from build123d import *

# Parameters (mm, degrees)
SKETCH_1_R      = 2.5
EXTRUDE_1_DEPTH = 140


with BuildPart() as part:
    # 草图1 → 凸台-拉伸1 (new, symmetric)
    with BuildSketch(Plane(origin=(0, 0, 0), x_dir=(1, 0, 0), z_dir=(0, 1, 0))):
        with BuildLine():
            Line((15.752176799, 53.551974455), (15.752176799, 48.473294799))
            Line((15.752176799, 48.473294799), (12.791516627, 45.512634627))
            Line((12.791516627, 45.512634627), (11.152176799, 45.512634627))
            Line((11.152176799, 45.512634627), (11.152176799, 47.912634627))
            Line((11.152176799, 47.912634627), (10.152176799, 47.912634627))
            Line((10.152176799, 47.912634627), (10.152176799, 47.412634627))
            Line((10.152176799, 47.412634627), (9.352176799, 47.412634627))
            Line((9.352176799, 47.412634627), (9.352176799, 42.512634627))
            ThreePointArc((9.352176799, 42.512634627), (9.791516627, 41.451974455), (10.852176799, 41.012634627))
            Line((10.852176799, 41.012634627), (15.752176799, 41.012634627))
            Line((15.752176799, 41.012634627), (15.752176799, 41.812634627))
            Line((15.752176799, 41.812634627), (16.252176799, 41.812634627))
            Line((16.252176799, 41.812634627), (16.252176799, 42.812634627))
            Line((16.252176799, 42.812634627), (13.852176799, 42.812634627))
            Line((13.852176799, 42.812634627), (13.852176799, 44.451974455))
            Line((13.852176799, 44.451974455), (16.812836971, 47.412634627))
            Line((16.812836971, 47.412634627), (21.891516627, 47.412634627))
            Line((21.891516627, 47.412634627), (24.852176799, 44.451974455))
            Line((24.852176799, 44.451974455), (24.852176799, 42.812634627))
            Line((24.852176799, 42.812634627), (22.452176799, 42.812634627))
            Line((22.452176799, 42.812634627), (22.452176799, 41.812634627))
            Line((22.452176799, 41.812634627), (22.952176799, 41.812634627))
            Line((22.952176799, 41.812634627), (22.952176799, 41.012634627))
            Line((22.952176799, 41.012634627), (27.852176799, 41.012634627))
            ThreePointArc((27.852176799, 41.012634627), (28.912836971, 41.451974455), (29.352176799, 42.512634627))
            Line((29.352176799, 42.512634627), (29.352176799, 47.412634627))
            Line((29.352176799, 47.412634627), (28.552176799, 47.412634627))
            Line((28.552176799, 47.412634627), (28.552176799, 47.912634627))
            Line((28.552176799, 47.912634627), (27.552176799, 47.912634627))
            Line((27.552176799, 47.912634627), (27.552176799, 45.512634627))
            Line((27.552176799, 45.512634627), (25.912836971, 45.512634627))
            Line((25.912836971, 45.512634627), (22.952176799, 48.473294799))
            Line((22.952176799, 48.473294799), (22.952176799, 53.551974455))
            Line((22.952176799, 53.551974455), (25.912836971, 56.512634627))
            Line((25.912836971, 56.512634627), (27.552176799, 56.512634627))
            Line((27.552176799, 56.512634627), (27.552176799, 54.112634627))
            Line((27.552176799, 54.112634627), (28.552176799, 54.112634627))
            Line((28.552176799, 54.112634627), (28.552176799, 54.612634627))
            Line((28.552176799, 54.612634627), (29.352176799, 54.612634627))
            Line((29.352176799, 54.612634627), (29.352176799, 59.512634627))
            ThreePointArc((29.352176799, 59.512634627), (28.912836971, 60.573294799), (27.852176799, 61.012634627))
            Line((27.852176799, 61.012634627), (22.952176799, 61.012634627))
            Line((22.952176799, 61.012634627), (22.952176799, 60.212634627))
            Line((22.952176799, 60.212634627), (22.452176799, 60.212634627))
            Line((22.452176799, 60.212634627), (22.452176799, 59.212634627))
            Line((22.452176799, 59.212634627), (24.852176799, 59.212634627))
            Line((24.852176799, 59.212634627), (24.852176799, 57.573294799))
            Line((24.852176799, 57.573294799), (21.891516627, 54.612634627))
            Line((21.891516627, 54.612634627), (16.812836971, 54.612634627))
            Line((16.812836971, 54.612634627), (13.852176799, 57.573294799))
            Line((13.852176799, 57.573294799), (13.852176799, 59.212634627))
            Line((13.852176799, 59.212634627), (16.252176799, 59.212634627))
            Line((16.252176799, 59.212634627), (16.252176799, 60.212634627))
            Line((16.252176799, 60.212634627), (15.752176799, 60.212634627))
            Line((15.752176799, 60.212634627), (15.752176799, 61.012634627))
            Line((15.752176799, 61.012634627), (10.852176799, 61.012634627))
            ThreePointArc((10.852176799, 61.012634627), (9.791516627, 60.573294799), (9.352176799, 59.512634627))
            Line((9.352176799, 59.512634627), (9.352176799, 54.612634627))
            Line((9.352176799, 54.612634627), (10.152176799, 54.612634627))
            Line((10.152176799, 54.612634627), (10.152176799, 54.112634627))
            Line((10.152176799, 54.112634627), (11.152176799, 54.112634627))
            Line((11.152176799, 54.112634627), (11.152176799, 56.512634627))
            Line((11.152176799, 56.512634627), (12.791516627, 56.512634627))
            Line((12.791516627, 56.512634627), (15.752176799, 53.551974455))
        make_face()
        with Locations(Location((19.352176799, 51.012634627, 0), (0, 0, 270))):
            Circle(SKETCH_1_R, mode=Mode.SUBTRACT)
    extrude(amount=EXTRUDE_1_DEPTH, both=True)


solid = part.part
Build history of the part. All positions in model axes, mm. A direction names the side the tool comes from. Coordinates: 2 decimals unless noted, no trailing zeros. Use CSV: the item, a comma, the result in double quotes. Start each with the question number.
Q1. Pull direction X, two halves, no side cores. Call faces 4 (the flat face through (19, 2, -47.413)), 5 (the flat face through (13, 2, -41.013)), 6 (the flat face through (29.352, 2, -45)): released by +X, released by -X, zero draft, split by the parting line, or undercut.
Q2. Drill centre lines: probe 1 along Z at (x, y) = (12.25, -97); probe 2 along Z at (x, y) = (19.5, 102); probe 3 along X at (y, z) = (109, -58.25). Where is each one in solid material? Low to high.
Q3. Flat gauge pins, fed straight in: pin 1 Ø0.9 at (x, y) = (9.5, -19.5) entering from +Z; pin 2 Ø1.5 at (x, y) = (22.5, -63) entering from -Z; pin 3 Ø0.6 at (x, y) = (10, 13.5) entering from -Z; pin 4 Ø0.9 at (y, z) = (10, -60.5) entering from +X. Where does each tip first touch, or does it go through?
Q4. 3-axis set-ups, long thin cutter, end or side, ignore diameter. For faces 1 (the flat face through (15.752, 2, -51)), 2 (the flat face through (19, 2, -54.613)), 3 (the flat face through (22.952, 2, -51)): which of +Z, -Z, +X, -X, +Y, -Y reach the whole face in a straight line?
Checked values:
1,face 4,"undercut"
1,face 5,"zero draft"
1,face 6,"released by +X"
2,probe 1,"z = -61.01 to -56.51, -45.51 to -41.01"
2,probe 2,"z = -54.61 to -53.51, -48.52 to -47.41"
2,probe 3,"x = 9.35 to 13.85, 24.85 to 29.35"
3,pin 1,"stops at z = -41.31"
3,pin 2,"stops at z = -61.01"
3,pin 3,"stops at z = -60.91"
3,pin 4,"stops at x = 29.25"
4,face 1,"-X, +Y, -Y"
4,face 2,"-Z, +Y, -Y"
4,face 3,"+X, +Y, -Y"
